The model under review builds one solid part; all positions refer to its coordinate system, in mm. Face numbers are marked on the shaded views. A direction names the side the tool comes from. Coordinates: 2 decimals unless noted, no trailing zeros. Order: outer loops, then holes, each group sorted by start corner. A loop starts at its lowest first (then second) coordinate and runs counter-clockwise, first axis right, second up. Notation, with made-up numbers: (-33.75, 87.5) -> (13.25, 87.5) arc R15 cw to (13.25, 107.5) -> close; hole circle Ø2 at (26, -34). An arc over 180 degrees is marked (long way). Use one line per item in the form item = value. Start each with the question number.
(1) Insertion check: pin 1 Ø4 at (x, y) = (-12.5, 36) entering from -Z; pin 2 Ø1 at (x, z) = (1, -0.5) entering from -Y; pin 3 Ø15.5 at (y, z) = (11.5, -7.5) entering from +X. Each pin has a flat end and moves straight along its axis. Give the tip position at first contact, or say it passes through.
(2) For the marked faces 1 and 2, list the 3-axis set-ups (+Z, -Z, +X, -X, +Y, -Y) from which the entire face can be reached by the end or side of a thin tool; tool diameter is ignored.
(3) Wall thickness on line 1 along X through (y, z) = (1.85, -11.2); line 2 along X through (y, z) = (6, -1.95); line 3 along Y through (x, z) = (-26.5, -0.55): over which ranges is each line inside the solid? List them lowest first.
(4) Take a section at C-C (z = 13.5). State the section outline as (x, y) points, then the cut area to 3 significant figures.
(5) Take a section at D-D (y = 35.5). State the section outline as (x, z) points, then the cut area to 3 significant figures.
(6) Take a section at A-A (y = 28.5). State the section outline as (x, z) points.
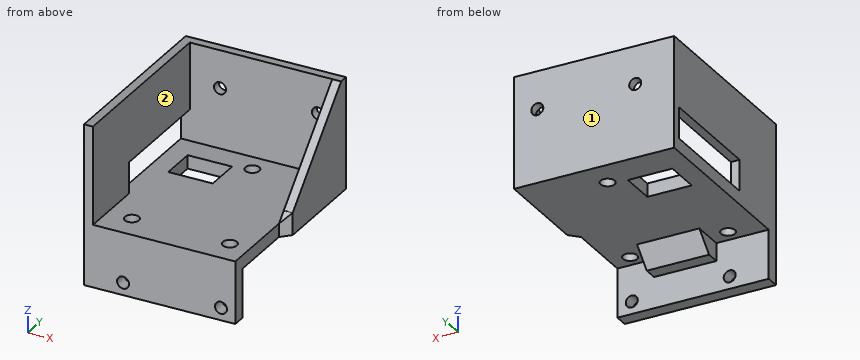
Autodesk Inventor part; units mm, degrees
ref_plane "YZ Plane" through (0, 0, 0) normal (1, 0, 0) x (0, 1, 0)
ref_plane "XZ Plane" through (0, 0, 0) normal (0, 1, 0) x (-1, 0, 0)
ref_plane "XY Plane" through (0, 0, 0) normal (0, 0, 1) x (1, 0, 0)
sketch "Sketch1" plane through (0, 0, 0) normal (0, 1, 0) x (-1, 0, 0)
  line L0 (0, 0) -> (34, 0)
  line L1 (34, 0) -> (34, -14)
  line L2 (34, -14) -> (0, -14)
  line L3 (0, -14) -> (0, 0)
  dimension "d0" = 34
  dimension "d1" = 14
extrude "Extrusion1" add sketch "Sketch1" along normal blind 3
sketch "Sketch2" plane through (0, 3, 0) normal (0, 1, 0) x (1, 0, 0)
  line L0 (-34, 0) -> (0, 0)
  line L1 (0, 0) -> (0, 14)
  line L2 (0, 14) -> (-34, 14)
  line L3 (-34, 14) -> (-34, 0)
  point P0 (-25.23, 11.2)
  point P1 (-3.23, 11.2)
  dimension "d59" = 22
  dimension "d60" = 8.77
hole "Hole1" at (-25.23, 3, -11.2) at (-3.23, 3, -11.2) direction (0, -1, 0) diameter 2.7 end through all
sketch "Sketch3" plane through (0, 3, 0) normal (0, 1, 0) x (1, 0, 0)
  circle A0 centre (-25.23, 11.2) radius 1.35
  circle A1 centre (-3.23, 11.2) radius 1.35
  line L0 (-34, 0) -> (0, 0)
  line L1 (0, 0) -> (0, 14)
  line L2 (0, 14) -> (-34, 14)
  line L3 (-34, 14) -> (-34, 0)
  line L4 (0, 0) -> (-34, 0)
  line L5 (-34, 0) -> (0, 0)
  line L6 (0, 0) -> (0, 3)
  line L7 (0, 3) -> (-34, 3)
  line L8 (-34, 3) -> (-34, 0)
  dimension "d14" = 3
extrude "Extrusion2" add sketch "Sketch3" along normal blind 39 contours L3 L7 L1 L0
sketch "Sketch4" plane through (0, 42, 0) normal (0, 1, 0) x (1, 0, 0)
  line L0 (-34, 0) -> (0, 0)
  line L1 (0, 0) -> (0, 3)
  line L2 (0, 3) -> (-34, 3)
  line L3 (-34, 3) -> (-34, 0)
  line L4 (-34, 3) -> (0, 3)
  line L5 (0, 3) -> (0, -22)
  line L6 (0, -22) -> (-34, -22)
  line L7 (-34, -22) -> (-34, 3)
  dimension "d17" = 25
extrude "Extrusion3" add sketch "Sketch4" against normal blind 2 contours L0 L5 L6 L7
sketch "Sketch6" plane through (0, 42, 0) normal (0, 1, 0) x (1, 0, 0)
  line L0 (0, -22) -> (0, 3)
  line L1 (0, 3) -> (-34, 3)
  line L2 (-34, 3) -> (-34, -22)
  line L3 (-34, -22) -> (0, -22)
  line L4 (0, 14) -> (0, -22)
  point P0 (0, 0)
  point P1 (-3.23, -13.5)
  point P2 (-25.23, -13.5)
  dimension "d57" = 22
  dimension "d58" = 3.23
hole "Hole2" at (-3.23, 42, 13.5) at (-25.23, 42, 13.5) direction (0, -1, 0) diameter 2.7 end through all
sketch "Sketch7" plane through (-34, 0, 0) normal (0, 0, 1) x (1, 0, 0)
  line L0 (34, 40) -> (0, 40)
  line L1 (0, 0) -> (0, 40)
  line L2 (34, 0) -> (0, 0)
  line L3 (34, 0) -> (34, 40)
  point P0 (7.5, 6)
  point P1 (29.5, 6)
  point P2 (18.5, 35.5)
  dimension "d50" = 11
  dimension "d51" = 29.5
  dimension "d52" = 22
  dimension "d55" = 4.5
hole "Hole3" at (-26.5, 6, 0) at (-4.5, 6, 0) at (-15.5, 35.5, 0) direction (0, 0, -1) diameter 3.2 end through all
sketch "Sketch8" plane through (-34, 0, 0) normal (0, 0, 1) x (1, 0, 0)
  circle A0 centre (29.5, 6) radius 1.6
  circle A1 centre (7.5, 6) radius 1.6
  circle A2 centre (18.5, 35.5) radius 1.6
  line L0 (34, 40) -> (0, 40)
  line L1 (0, 0) -> (0, 40)
  line L2 (34, 0) -> (0, 0)
  line L3 (14.5, 34.5) -> (4.5, 34.5)
  line L4 (4.5, 34.5) -> (4.5, 26.5)
  line L5 (4.5, 26.5) -> (14.5, 26.5)
  line L6 (14.5, 26.5) -> (14.5, 34.5)
  line L7 (34, 0) -> (34, 40)
  dimension "d46" = 10
  dimension "d47" = 8
  dimension "d53" = 1
  dimension "d54" = 4
extrude "Extrusion5" cut sketch "Sketch8" against normal blind 3 contours L6 L5 L4 L3
sketch "Sketch9" plane through (-34, 0, -14) normal (-1, 0, 0) x (0, 0, 1)
  line L0 (14, 0) -> (0, 0)
  line L1 (14, 0) -> (14, 40)
  line L2 (36, 40) -> (14, 40)
  line L3 (36, 42) -> (36, 40)
  line L4 (11, 42) -> (36, 42)
  line L5 (11, 3) -> (11, 42)
  line L6 (0, 3) -> (11, 3)
  line L7 (0, 0) -> (0, 3)
  line L8 (14, 40) -> (36, 40)
  line L9 (36, 40) -> (36, 0)
  line L10 (36, 0) -> (14, 0)
  line L11 (14, 0) -> (14, 40)
extrude "Extrusion6" add sketch "Sketch9" against normal blind 2 contours L1 L2 L9 L10
sketch "Sketch10" plane through (0, 0, 0) normal (1, 0, 0) x (0, 0, -1)
  line L0 (14, 0) -> (0, 0)
  line L1 (14, 0) -> (14, 3)
  line L2 (3, 3) -> (14, 3)
  line L3 (3, 3) -> (3, 42)
  line L4 (-22, 42) -> (3, 42)
  line L5 (-22, 42) -> (-22, 40)
  line L6 (0, 40) -> (-22, 40)
  line L7 (0, 0) -> (0, 40)
  line L8 (-22, 42) -> (-22, 40)
  line L9 (3, 3) -> (3, 42)
  line L10 (-22, 42) -> (3, 42)
  line L11 (3, 42) -> (3, 20)
  line L12 (3, 20) -> (-22, 20)
  line L13 (-22, 20) -> (-22, 42)
  dimension "d63" = 22
extrude "Extrusion7" add sketch "Sketch10" along normal blind 2 contours L12 L13 L6 L7 | L7 L6 L5 L4 L3 L12
chamfer "Chamfer1" distance 2 angle 45 1 edges at (0, 20, -1.5)
chamfer "Chamfer2" distance 20 angle 45 1 edges at (1, 20, 22)
chamfer "Chamfer3" distance 1.99 angle 45 1 edges at (0.9999, 20, 0)
sketch "Sketch11" plane through (-34, 0, -14) normal (-1, 0, 0) x (0, 0, 1)
  line L0 (14, 40) -> (14, 0)
  line L1 (36, 40) -> (14, 40)
  line L2 (14, 40) -> (21, 40)
  line L3 (21, 40) -> (21, 15)
  line L4 (21, 15) -> (14, 15)
  line L5 (14, 15) -> (14, 40)
  dimension "d75" = 7
  dimension "d76" = 25
extrude "Extrusion8" cut sketch "Sketch11" against normal blind 2
sketch "Sketch12" plane through (0, 3, 0) normal (0, 1, 0) x (1, 0, 0)
  line L0 (-34, 3) -> (0, 3)
  line L1 (0, 3) -> (0, 14)
  line L2 (0, 14) -> (-34, 14)
  line L3 (-34, 14) -> (-34, 3)
  circle A0 centre (-25.23, 11.2) radius 1.35
  circle A1 centre (-3.23, 11.2) radius 1.35
  line L4 (-34, 3) -> (0, 3)
  line L5 (-3.23, 11.2) -> (-8.23, 11.2)
  line L6 (-8.23, 11.2) -> (-8.23, 3)
  line L7 (-8.23, 3) -> (-3.23, 3)
  line L8 (-3.23, 3) -> (-3.23, 11.2)
  line L9 (-25.23, 11.2) -> (-22.23, 11.2)
  line L10 (-22.23, 11.2) -> (-22.23, 3)
  line L11 (-22.23, 3) -> (-25.23, 3)
  line L12 (-25.23, 3) -> (-25.23, 11.2)
  line L13 (-8.23, 3) -> (-22.23, 3)
  line L14 (-22.23, 3) -> (-22.23, 7)
  line L15 (-22.23, 7) -> (-8.23, 7)
  line L16 (-8.23, 7) -> (-8.23, 3)
  point P0 (0, 0)
  dimension "d79" = 5
  dimension "d80" = 3
  dimension "d81" = 4
extrude "Extrusion9" add sketch "Sketch12" along normal blind 7 contours L10 L15 L6 L0
chamfer "Chamfer4" distance 4 angle 45 1 edges at (-15.23, 10, -7)
properties part number "PantatKanan" material "Iron, Gray"
Findings:
q1.pin_1 = -3
q1.pin_2 = 18.5
q1.pin_3 = 0
q2.face_1 = +Z, -Z, +X, -X, +Y
q2.face_2 = +Z, -Y
q3.line_1 = -34 to -26.58, -23.88 to -4.58, -1.88 to 0
q3.line_2 = -34 to -28.1, -24.9 to -6.1, -2.9 to 0
q3.line_3 = 0 to 4.4, 7.6 to 26.5, 34.5 to 42
q4.outline = (-34, 0) -> (-32, 0) -> (-32, 40) -> (-26.58, 40) -> (-26.58, 42) -> (-34, 42) -> close; (-23.88, 40) -> (-4.58, 40) -> (-4.58, 42) -> (-23.88, 42) -> close; (-1.88, 40) -> (0, 40) -> (0, 31.5) -> (2, 31.5) -> (2, 42) -> (-1.88, 42) -> close
q4.area = 158 mm²
q5.outline = (-34, -3) -> (-17.1, -3) -> (-17.1, 0) -> (-34, 0) -> close; (-34, 7) -> (-32, 7) -> (-32, 22) -> (-34, 22) -> close; (-13.9, -3) -> (2, -3) -> (2, 17.5) -> (0, 17.5) -> (0, 0) -> (-13.9, 0) -> close
q5.area = 163 mm²
q6.outline = (-34, -3) -> (-29.5, -3) -> (-29.5, 0) -> (-34, 0) -> close; (-34, 7) -> (-32, 7) -> (-32, 22) -> (-34, 22) -> close; (-19.5, -3) -> (2, -3) -> (2, 10.5) -> (0, 10.5) -> (0, 0) -> (-19.5, 0) -> close
